```python
from build123d import *

# Parameters (mm, degrees)
F0_W     = 12.7
F0_H     = 5.08
F1_DEPTH = 1.778
F3_W     = 3.957054
F3_H     = 2.032
F4_DEPTH = 10.16
F5_R     = 1.27
F6_DEPTH = 12.7


with BuildPart() as f1:
    # F0 (on Top) → F1 (new body)
    with BuildSketch(Plane.XY):
        Rectangle(F0_W, F0_H)
    extrude(amount=F1_DEPTH)

    # F3 (on offset) → F4 (join)
    with BuildSketch(Plane.XY.offset(1.778)):
        Rectangle(F3_W, F3_H)
    extrude(amount=F4_DEPTH)

    # F5 (on Front) → F6 (join)
    with BuildSketch(Plane.XZ):
        with Locations((0, 10.315562)):
            Circle(F5_R)
    extrude(amount=F6_DEPTH)


solid = f1.part
```
Geometry: final body of the model. Coordinates: model frame, mm. A direction names the side the tool comes from. Round coordinates to 2 decimals unless told otherwise and drop trailing zeros. Order: outer loops, then holes, each group sorted by start corner. A loop starts at its lowest first (then second) coordinate and runs counter-clockwise, first axis right, second up. Notation, with made-up numbers: (5.25, 23) -> (62.25, 23) arc R31 cw to (62.25, 50) -> close; hole circle Ø4 at (28, 36). An arc over 180 degrees is marked (long way). Use one line per item in the form item = value. Start each with the question number.
1. Cut plane D-D (z = 1.5). Return the cut outline in (x, y).
2. Cut plane A-A (x = 0). Return the cut outline in (y, z), then the cut area to 3 significant figures.
3. Pin query (flat end, axial travel): pin 1 Ø3 at (x, y) = (-2, -3.5) entering from +Z; pin 2 Ø4 at (x, y) = (-5, -2) entering from +Z; pin 3 Ø1.4 at (x, z) = (0, 1) entering from -Y. Return the tip coordinate at first contact, or that it passes through.
4. Reachability of faces 4 (the face through (0, 1.016, 7)), 5 (the face through (1.979, 0, 7)), 6 (the face through (0.59, -6.78, 9.19)), 7 (the face through (-1.979, 0, 7)) from +Z, -Z, +X, -X, +Y, -Y: full face, straight path, thin tool, end or side. Return the list, or none.
5. Cut plane B-B (z = 8.5). Return the cut outline in (x, y), then the cut area to 3 significant figures.
6. Cut plane C-C (y = -4.75). Return the cut outline in (x, z).
7. Draft query along Z for faces 1 (the face through (0, 2.54, 1)), 2 (the face through (0, 0, 0)), 3 (the face through (0, -1.016, 7)). Return one class per face: pulls with the +Z half, pulls with the -Z half, needs draft (parallel to the pull), parting line crosses it, or undercut.
8. Line query: probe 1 along Y at (x, z) = (3, 0.5); probe 2 along Z at (x, y) = (-5.5, -1.5); probe 3 along X at (y, z) = (-0.75, 8.75). Output: solid intervals per line, ascending.
Solution:
q1.outline = (-6.35, -2.54) -> (6.35, -2.54) -> (6.35, 2.54) -> (-6.35, 2.54) -> close
q2.outline = (-12.7, 9.05) -> (-1.02, 9.05) -> (-1.02, 1.78) -> (-2.54, 1.78) -> (-2.54, 0) -> (2.54, 0) -> (2.54, 1.78) -> (1.02, 1.78) -> (1.02, 11.94) -> (-1.02, 11.94) -> (-1.02, 11.59) -> (-12.7, 11.59) -> close
q2.area = 59.4 mm^2
q3.pin_1 = 11.48
q3.pin_2 = 1.78
q3.pin_3 = -2.54
q4.face_4 = +Z, +X, -X, +Y
q4.face_5 = +Z, +X, +Y, -Y
q4.face_6 = -Y
q4.face_7 = +Z, -X, +Y, -Y
q5.outline = (-1.98, -1.02) -> (1.98, -1.02) -> (1.98, 1.02) -> (-1.98, 1.02) -> close
q5.area = 8.04 mm^2
q6.outline = circle Ø2.54 at (0, 10.32)
q7.face_1 = needs draft
q7.face_2 = pulls with the -Z half
q7.face_3 = undercut
q8.probe_1 = -2.54 to 2.54
q8.probe_2 = 0 to 1.78
q8.probe_3 = -1.98 to 1.98
